from build123d import *

# Parameters (mm, degrees)
SKETCH_1_R          = 2
EXTRUDE_1_DEPTH     = 4
EXTRUDE_3_DEPTH     = 4
SKETCH_7_R          = 2
CUT_EXTRUDE_2_DEPTH = 10


with BuildPart() as part:
    # 草图1 → 凸台-拉伸1 (new body)
    with BuildSketch(Plane.XY):
        with BuildLine():
            Line((-180.694062755, -12.410089261), (126.305937245, -12.410089261))
            ThreePointArc((126.305937245, -12.410089261), (129.13436437, -11.238516386), (130.305937245, -8.410089261))
            Line((130.305937245, -8.410089261), (130.305937245, 7.71191214))
            Line((130.305937245, 7.71191214), (130.305937245, 17.589910739))
            Line((130.305937245, 17.589910739), (130.305937245, 39.589910739))
            ThreePointArc((130.305937245, 39.589910739), (129.13436437, 42.418337863), (126.305937245, 43.589910739))
            Line((126.305937245, 43.589910739), (-23.194062755, 43.589910739))
            ThreePointArc((-23.194062755, 43.589910739), (-26.022489879, 42.418337863), (-27.194062755, 39.589910739))
            Line((-27.194062755, 39.589910739), (-27.194062755, 27.589910739))
            ThreePointArc((-27.194062755, 27.589910739), (-30.122994943, 20.518842927), (-37.194062755, 17.589910739))
            Line((-37.194062755, 17.589910739), (-180.694062755, 17.589910739))
            ThreePointArc((-180.694062755, 17.589910739), (-183.522489879, 16.418337863), (-184.694062755, 13.589910739))
            Line((-184.694062755, 13.589910739), (-184.694062755, -8.410089261))
            ThreePointArc((-184.694062755, -8.410089261), (-183.522489879, -11.238516386), (-180.694062755, -12.410089261))
        make_face()
        with Locations((-127.194062755, -7.410089261)):
            Circle(SKETCH_1_R, mode=Mode.SUBTRACT)
        with Locations((-88.864062755, -7.410089261)):
            Circle(SKETCH_1_R, mode=Mode.SUBTRACT)
        with Locations((34.475937245, -7.410089261)):
            Circle(SKETCH_1_R, mode=Mode.SUBTRACT)
        with Locations((72.805937245, -7.410089261)):
            Circle(SKETCH_1_R, mode=Mode.SUBTRACT)
        with Locations((34.475937245, 38.589910739)):
            Circle(SKETCH_1_R, mode=Mode.SUBTRACT)
        with Locations((122.805937245, 31.589910739)):
            Circle(SKETCH_1_R, mode=Mode.SUBTRACT)
        with Locations((72.805937245, 38.589910739)):
            Circle(SKETCH_1_R, mode=Mode.SUBTRACT)
    extrude(amount=EXTRUDE_1_DEPTH)

    # 草图2 → 凸台-拉伸3 (add)
    with BuildSketch(Plane(origin=(0, 0, 0), x_dir=(-1, 0, 0), z_dir=(0, 0, -1))):
        with BuildLine():
            Line((53.194062755, 43.589910739), (23.194062755, 43.589910739))
            Line((23.194062755, 43.589910739), (23.194062755, 17.589910739))
            Line((23.194062755, 17.589910739), (57.194062755, 17.589910739))
            Line((57.194062755, 17.589910739), (61.194062755, 17.589910739))
            ThreePointArc((61.194062755, 17.589910739), (58.36563563, 18.761483614), (57.194062755, 21.589910739))
            Line((57.194062755, 21.589910739), (57.194062755, 39.589910739))
            ThreePointArc((57.194062755, 39.589910739), (56.022489879, 42.418337863), (53.194062755, 43.589910739))
        make_face()
    extrude(amount=-EXTRUDE_3_DEPTH)

    # 草图7 → 切除-拉伸2 (cut)
    with BuildSketch(Plane(origin=(0, 0, 0), x_dir=(-1, 0, 0), z_dir=(0, 0, -1))):
        with Locations((29.194062755, 32.589910739)):
            Circle(SKETCH_7_R)
    extrude(amount=-CUT_EXTRUDE_2_DEPTH, mode=Mode.SUBTRACT)


solid = part.part
Geometry check sheet. Reference: the model listing, model coordinates, mm. Give positions to 0.01 mm unless a question says otherwise; leave off trailing zeros. Answer as a JSON object with one key per item and string values. Group by question number.
Item 1: Sectioned sample at A-A on z = 0.65. Give the number of separate pieces and of enclosed holes in the cut face, plus the area to 3 significant figures.
Item 2: Gauge pin test, flat end, axial feed: pin 1 (1.2 mm diameter, centred on x = -119, z = 2, fed in from +Y). Record the tip position at first contact, or that the pin passes through.
Item 3: Material ranges on L1, parallel to X at y = -8, z = 0.65; L2, parallel to Y at x = -97, z = 3.1; L3, parallel to X at y = 24.5, z = 0.35, recorded low to high.
Findings below:
{
 "1": {"separate pieces": "1", "enclosed holes": "8", "area": "14,200 mm2"},
 "2": {"pin 1": "y = 17.59"},
 "3": {"L1": "-184.69 to -129.11, -125.28 to -90.78, -86.95 to 32.56, 36.39 to 70.89, 74.72 to 130.31", "L2": "-12.41 to 17.59", "L3": "-57.19 to 130.31"}
}
